Source: CAD feature listing. Evaluate the final solid. Frame: model axes, mm. Face numbers are marked on the shaded views. A direction names the side the tool comes from. Coordinates: 2 decimals unless noted, no trailing zeros. Loops run counter-clockwise (first coordinate to the right, second up) from the corner with the lowest first, then second, coordinate; pieces in that order, holes last.
Item 1: Reachability of the marked faces 1, 2, 3 and 4 from +Z, -Z, +X, -X, +Y, -Y: full face, straight path, thin tool, end or side. Return the list, or none.
Item 2: Section query A-A, the plane z = 19.5. Return the cut outline in (x, y).
Item 3: Line query: probe 1 along Z at (x, y) = (34.5, -25); probe 2 along X at (y, z) = (77, 20); probe 3 along X at (y, z) = (-0.5, 20.5). Output: solid intervals per line, ascending.
Item 4: Pin query (flat end, axial travel): pin 1 Ø6 at (y, z) = (73, 20.5) entering from -X; pin 2 Ø7.5 at (x, z) = (-9, 22.5) entering from -Y; pin 3 Ø5 at (y, z) = (-30.5, 9.5) entering from -X. Return the tip coordinate at first contact, or that it passes through.
Item 5: Section query B-B, the plane z = 2.5. Return the cut outline in (x, y), then the cut area to 3 significant figures.
Item 6: Pull-direction query (Y, two-part tool) for the marked faces 5, 6 and 7; classes: +Y half, -Y half, draft (parallel to the pull), parting line (faces both ways), or undercut.
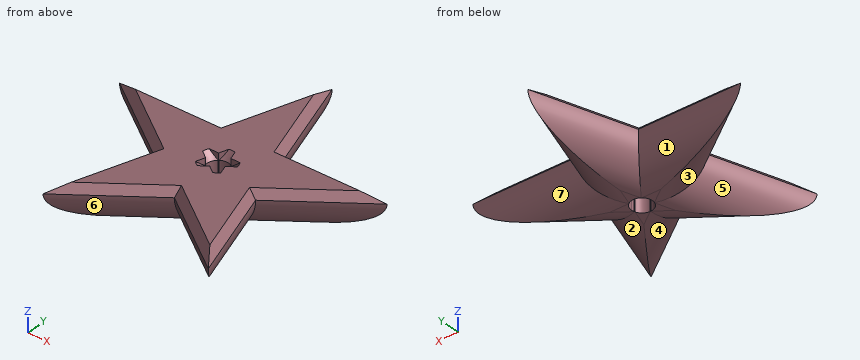
```python
from build123d import *

# Parameters (mm, degrees)
F1_DEPTH     = 30
F2_SIZE      = 5
F3_R         = 24.99999
F5_DEPTH     = 35
F6_T4_ANGLE  = 264.2993733481
F6_T11_ANGLE = 264.2993733481
F6_T18_ANGLE = 264.2993733481
F6_T24_ANGLE = 264.2993733481
F6_T30_ANGLE = 264.2993733481
F6_T37_ANGLE = 264.2993733481
F6_T44_ANGLE = 264.2993733481
F6_T51_ANGLE = 264.2993733481
F6_T57_ANGLE = 264.2993733481
F6_T63_ANGLE = 264.2993733481
F6_T70_ANGLE = 264.299373348
F6_T77_ANGLE = 264.299373348
F6_T84_ANGLE = 264.299373348


# Not quite as in the source:
# - a fillet or chamfer that OpenCascade refuses, or shapes differently, is made with other operations: its cross-section is extruded or revolved along the edge and cut away or added
# - a fillet or chamfer is up to 0.001 mm smaller than in the source, because OpenCascade refuses the exact size


with BuildPart() as f1:
    # F0 (on Top) → F1 (new body)
    with BuildSketch(Plane.XY):
        Polygon((22.451398829, 30.9016994375), (0, 100), (-22.451398829, 30.9016994375), (-95.1056516295, 30.9016994375), (-36.3271264003, -11.803398875), (-58.7785252292, -80.9016994375), (0, -38.196601125), (58.7785252292, -80.9016994375), (36.3271264003, -11.803398875), (95.1056516295, 30.9016994375), align=None)
    extrude(amount=F1_DEPTH)

    # F2
    f2_edges = [f1.edges().sort_by_distance(p)[0] for p in [
        (65.716389, 9.54915, 30),
        (58.778525, 30.901699, 30),
        (11.225699, 65.45085, 30),
        (-11.225699, 65.45085, 30),
        (-58.778525, 30.901699, 30),
        (-65.716389, 9.54915, 30),
        (-47.552826, -46.352549, 30),
        (-29.389263, -59.54915, 30),
        (29.389263, -59.54915, 30),
        (47.552826, -46.352549, 30),
    ]]
    chamfer(f2_edges, length=F2_SIZE)

    # F3 (radius 25 in the source; OpenCascade refuses exactly that, so slightly less here)
    f3_edges = [f1.edges().sort_by_distance(p)[0] for p in [
        (65.716389, 9.54915, 0),
        (58.778525, 30.901699, 0),
        (11.225699, 65.45085, 0),
        (-11.225699, 65.45085, 0),
        (-58.778525, 30.901699, 0),
        (-65.716389, 9.54915, 0),
        (-47.552826, -46.352549, 0),
        (-29.389263, -59.54915, 0),
        (29.389263, -59.54915, 0),
        (47.552826, -46.352549, 0),
    ]]
    fillet(f3_edges, radius=F3_R)

    # F4 (on face) → F5 (cut)
    with BuildSketch(Plane(origin=(0, 0, 0), x_dir=(1, 0, 0), z_dir=(0, 0, -1))):
        with BuildLine():
            ThreePointArc((4.6281557575, -5.9017094375), (6.7439294251, -3.2816788249), (7.5, 0))
            ThreePointArc((7.5, 0), (7.4279525521, 1.0370732295), (7.2131944311, 2.0542215312))
            Line((7.2131944311, 2.0542215312), (6.9378755413, 2.2542524134))
            Line((6.9378755413, 2.2542524134), (7.0430379995, 2.5779091795))
            ThreePointArc((7.0430379995, 2.5779091795), (4.4083893922, 6.0676274578), (0.2753188897, 7.4949449303))
            Line((0.2753188897, 7.4949449303), (0, 7.2949140482))
            Line((0, 7.2949140482), (-0.2753188897, 7.4949449303))
            ThreePointArc((-0.2753188897, 7.4949449303), (-4.4083893922, 6.0676274578), (-7.0430379995, 2.5779091795))
            Line((-7.0430379995, 2.5779091795), (-6.9378755413, 2.2542524134))
            Line((-6.9378755413, 2.2542524134), (-7.2131944311, 2.0542215312))
            ThreePointArc((-7.2131944311, 2.0542215312), (-7.1329238722, -2.3176274578), (-4.6281557575, -5.9017094375))
            Line((-4.6281557575, -5.9017094375), (-4.2878428943, -5.9017094375))
            Line((-4.2878428943, -5.9017094375), (-4.1826804361, -6.2253662036))
            ThreePointArc((-4.1826804361, -6.2253662036), (0, -7.5), (4.1826804361, -6.2253662036))
            Line((4.1826804361, -6.2253662036), (4.2878428943, -5.9017094375))
            Line((4.2878428943, -5.9017094375), (4.6281557575, -5.9017094375))
        make_face()
    extrude(amount=-F5_DEPTH, mode=Mode.SUBTRACT)

    # F6: chamfer of 5 on 5 edges, made by hand


with BuildPart() as f6_tool2:
    # F6_s3 → F6_t4 (revolve)
    with BuildSketch(Plane(origin=(0, 0, 0), x_dir=(0, 0, 1), z_dir=(0.9124797315, 0.4091219129, 0))):
        Polygon((30, 12.5), (25, 7.5), (30, 7.5), align=None)
    revolve(axis=Axis((0, 0, 30), (0, 0, -1)), revolution_arc=F6_T4_ANGLE)

    split(bisect_by=Plane(origin=(-5.6128592178, 1.823728512, 0), x_dir=(0, 0, 1), z_dir=(0.9510565163, -0.3090169944, 0)), keep=Keep.TOP)

    split(bisect_by=Plane(origin=(-3.4689377707, -4.7745832308, 0), x_dir=(0, 0, 1), z_dir=(0.5877852523, 0.8090169944, 0)), keep=Keep.TOP)

    split(bisect_by=Plane(origin=(5.6128592178, 1.823728512, 0), x_dir=(0, 0, 1), z_dir=(-0.9510565163, -0.3090169944, 0)), keep=Keep.TOP)


with BuildPart() as f1_1:
    add(f1.part)

    # F6_t1: cut F6_tool2
    add(f6_tool2.part, mode=Mode.SUBTRACT)


with BuildPart() as f6_tool9:
    # F6_s10 → F6_t11 (revolve)
    with BuildSketch(Plane(origin=(0, 0, 0), x_dir=(0, 0, 1), z_dir=(0.9124797315, 0.4091219129, 0))):
        Polygon((30, 12.5), (25, 7.5), (30, 7.5), align=None)
    revolve(axis=Axis((0, 0, 30), (0, 0, -1)), revolution_arc=F6_T11_ANGLE)

    split(bisect_by=Plane.XZ.offset(-5.9017094375), keep=Keep.TOP)

    split(bisect_by=Plane(origin=(-5.6128592178, 1.823728512, 0), x_dir=(0, 0, 1), z_dir=(0.9510565163, -0.3090169944, 0)), keep=Keep.TOP)

    split(bisect_by=Plane(origin=(3.4689377707, -4.7745832308, 0), x_dir=(0, 0, 1), z_dir=(-0.5877852523, 0.8090169944, 0)), keep=Keep.TOP)


with BuildPart() as f1_2:
    add(f1_1.part)

    # F6_t8: cut F6_tool9
    add(f6_tool9.part, mode=Mode.SUBTRACT)


with BuildPart() as f6_tool16:
    # F6_s17 → F6_t18 (revolve)
    with BuildSketch(Plane(origin=(0, 0, 0), x_dir=(0, 0, 1), z_dir=(0.9124797315, 0.4091219129, 0))):
        Polygon((30, 12.5), (25, 7.5), (30, 7.5), align=None)
    revolve(axis=Axis((0, 0, 30), (0, 0, -1)), revolution_arc=F6_T18_ANGLE)

    split(bisect_by=Plane.XZ.offset(-5.9017094375), keep=Keep.TOP)

    split(bisect_by=Plane(origin=(-3.4689377707, -4.7745832308, 0), x_dir=(0, 0, 1), z_dir=(0.5877852523, 0.8090169944, 0)), keep=Keep.TOP)


with BuildPart() as f1_3:
    add(f1_2.part)

    # F6_t15: cut F6_tool16
    add(f6_tool16.part, mode=Mode.SUBTRACT)


with BuildPart() as f6_tool22:
    # F6_s23 → F6_t24 (revolve)
    with BuildSketch(Plane(origin=(0, 0, 0), x_dir=(0, 0, 1), z_dir=(0.6710698053, -0.7413941707, 0))):
        Polygon((30, 12.5), (25, 7.5), (30, 7.5), align=None)
    revolve(axis=Axis((0, 0, 30), (0, 0, -1)), revolution_arc=F6_T24_ANGLE)

    split(bisect_by=Plane(origin=(5.6128592178, 1.823728512, 0), x_dir=(0, 0, 1), z_dir=(-0.9510565163, -0.3090169944, 0)), keep=Keep.TOP)

    split(bisect_by=Plane(origin=(-5.6128592178, 1.823728512, 0), x_dir=(0, 0, 1), z_dir=(0.9510565163, -0.3090169944, 0)), keep=Keep.TOP)


with BuildPart() as f1_4:
    add(f1_3.part)

    # F6_t21: cut F6_tool22
    add(f6_tool22.part, mode=Mode.SUBTRACT)


with BuildPart() as f6_tool28:
    # F6_s29 → F6_t30 (revolve)
    with BuildSketch(Plane(origin=(0, 0, 0), x_dir=(0, 0, 1), z_dir=(0.6710698053, -0.7413941707, 0))):
        Polygon((30, 12.5), (25, 7.5), (30, 7.5), align=None)
    revolve(axis=Axis((0, 0, 30), (0, 0, -1)), revolution_arc=F6_T30_ANGLE)

    split(bisect_by=Plane(origin=(3.4689377707, -4.7745832308, 0), x_dir=(0, 0, 1), z_dir=(-0.5877852523, 0.8090169944, 0)), keep=Keep.TOP)

    split(bisect_by=Plane.XZ.offset(-5.9017094375), keep=Keep.TOP)

    split(bisect_by=Plane(origin=(-3.4689377707, -4.7745832308, 0), x_dir=(0, 0, 1), z_dir=(0.5877852523, 0.8090169944, 0)), keep=Keep.TOP)


with BuildPart() as f1_5:
    add(f1_4.part)

    # F6_t27: cut F6_tool28
    add(f6_tool28.part, mode=Mode.SUBTRACT)


with BuildPart() as f6_tool35:
    # F6_s36 → F6_t37 (revolve)
    with BuildSketch(Plane(origin=(0, 0, 0), x_dir=(0, 0, 1), z_dir=(-0.497735783, -0.8673287095, 0))):
        Polygon((30, 12.5), (25, 7.5), (30, 7.5), align=None)
    revolve(axis=Axis((0, 0, 30), (0, 0, -1)), revolution_arc=F6_T37_ANGLE)

    split(bisect_by=Plane(origin=(5.6128592178, 1.823728512, 0), x_dir=(0, 0, 1), z_dir=(-0.9510565163, -0.3090169944, 0)), keep=Keep.TOP)

    split(bisect_by=Plane.XZ.offset(-5.9017094375), keep=Keep.TOP)

    split(bisect_by=Plane(origin=(-3.4689377707, -4.7745832308, 0), x_dir=(0, 0, 1), z_dir=(0.5877852523, 0.8090169944, 0)), keep=Keep.TOP)


with BuildPart() as f1_6:
    add(f1_5.part)

    # F6_t34: cut F6_tool35
    add(f6_tool35.part, mode=Mode.SUBTRACT)


with BuildPart() as f6_tool42:
    # F6_s43 → F6_t44 (revolve)
    with BuildSketch(Plane(origin=(0, 0, 0), x_dir=(0, 0, 1), z_dir=(-0.497735783, -0.8673287095, 0))):
        Polygon((30, 12.5), (25, 7.5), (30, 7.5), align=None)
    revolve(axis=Axis((0, 0, 30), (0, 0, -1)), revolution_arc=F6_T44_ANGLE)

    split(bisect_by=Plane(origin=(3.4689377707, -4.7745832308, 0), x_dir=(0, 0, 1), z_dir=(-0.5877852523, 0.8090169944, 0)), keep=Keep.TOP)

    split(bisect_by=Plane(origin=(5.6128592178, 1.823728512, 0), x_dir=(0, 0, 1), z_dir=(-0.9510565163, -0.3090169944, 0)), keep=Keep.TOP)

    split(bisect_by=Plane(origin=(-5.6128592178, 1.823728512, 0), x_dir=(0, 0, 1), z_dir=(0.9510565163, -0.3090169944, 0)), keep=Keep.TOP)


with BuildPart() as f1_7:
    add(f1_6.part)

    # F6_t41: cut F6_tool42
    add(f6_tool42.part, mode=Mode.SUBTRACT)


with BuildPart() as f6_tool49:
    # F6_s50 → F6_t51 (revolve)
    with BuildSketch(Plane(origin=(0, 0, 0), x_dir=(0, 0, 1), z_dir=(-0.497735783, -0.8673287095, 0))):
        Polygon((30, 12.5), (25, 7.5), (30, 7.5), align=None)
    revolve(axis=Axis((0, 0, 30), (0, 0, -1)), revolution_arc=F6_T51_ANGLE)

    split(bisect_by=Plane(origin=(3.4689377707, -4.7745832308, 0), x_dir=(0, 0, 1), z_dir=(-0.5877852523, 0.8090169944, 0)), keep=Keep.TOP)

    split(bisect_by=Plane.XZ.offset(-5.9017094375), keep=Keep.TOP)


with BuildPart() as f1_8:
    add(f1_7.part)

    # F6_t48: cut F6_tool49
    add(f6_tool49.part, mode=Mode.SUBTRACT)


with BuildPart() as f6_tool55:
    # F6_s56 → F6_t57 (revolve)
    with BuildSketch(Plane(origin=(0, 0, 0), x_dir=(0, 0, 1), z_dir=(-0.9786874366, 0.2053555488, 0))):
        Polygon((30, 12.5), (25, 7.5), (30, 7.5), align=None)
    revolve(axis=Axis((0, 0, 30), (0, 0, -1)), revolution_arc=F6_T57_ANGLE)

    split(bisect_by=Plane(origin=(5.6128592178, 1.823728512, 0), x_dir=(0, 0, 1), z_dir=(-0.9510565163, -0.3090169944, 0)), keep=Keep.TOP)

    split(bisect_by=Plane(origin=(-3.4689377707, -4.7745832308, 0), x_dir=(0, 0, 1), z_dir=(0.5877852523, 0.8090169944, 0)), keep=Keep.TOP)


with BuildPart() as f1_9:
    add(f1_8.part)

    # F6_t54: cut F6_tool55
    add(f6_tool55.part, mode=Mode.SUBTRACT)


with BuildPart() as f6_tool61:
    # F6_s62 → F6_t63 (revolve)
    with BuildSketch(Plane(origin=(0, 0, 0), x_dir=(0, 0, 1), z_dir=(-0.9786874366, 0.2053555488, 0))):
        Polygon((30, 12.5), (25, 7.5), (30, 7.5), align=None)
    revolve(axis=Axis((0, 0, 30), (0, 0, -1)), revolution_arc=F6_T63_ANGLE)

    split(bisect_by=Plane(origin=(3.4689377707, -4.7745832308, 0), x_dir=(0, 0, 1), z_dir=(-0.5877852523, 0.8090169944, 0)), keep=Keep.TOP)

    split(bisect_by=Plane.XZ.offset(-5.9017094375), keep=Keep.TOP)

    split(bisect_by=Plane(origin=(-5.6128592178, 1.823728512, 0), x_dir=(0, 0, 1), z_dir=(0.9510565163, -0.3090169944, 0)), keep=Keep.TOP)


with BuildPart() as f1_10:
    add(f1_9.part)

    # F6_t60: cut F6_tool61
    add(f6_tool61.part, mode=Mode.SUBTRACT)


with BuildPart() as f6_tool68:
    # F6_s69 → F6_t70 (revolve)
    with BuildSketch(Plane(origin=(0, 0, 0), x_dir=(0, 0, 1), z_dir=(-0.1071263172, 0.9942454185, 0))):
        Polygon((30, 12.5), (25, 7.5), (30, 7.5), align=None)
    revolve(axis=Axis((0, 0, 30), (0, 0, -1)), revolution_arc=F6_T70_ANGLE)

    split(bisect_by=Plane(origin=(3.4689377707, -4.7745832308, 0), x_dir=(0, 0, 1), z_dir=(-0.5877852523, 0.8090169944, 0)), keep=Keep.TOP)

    split(bisect_by=Plane(origin=(-3.4689377707, -4.7745832308, 0), x_dir=(0, 0, 1), z_dir=(0.5877852523, 0.8090169944, 0)), keep=Keep.TOP)

    split(bisect_by=Plane.XZ.offset(-5.9017094375), keep=Keep.TOP)


with BuildPart() as f1_11:
    add(f1_10.part)

    # F6_t67: cut F6_tool68
    add(f6_tool68.part, mode=Mode.SUBTRACT)


with BuildPart() as f6_tool75:
    # F6_s76 → F6_t77 (revolve)
    with BuildSketch(Plane(origin=(0, 0, 0), x_dir=(0, 0, 1), z_dir=(-0.1071263172, 0.9942454185, 0))):
        Polygon((30, 12.5), (25, 7.5), (30, 7.5), align=None)
    revolve(axis=Axis((0, 0, 30), (0, 0, -1)), revolution_arc=F6_T77_ANGLE)

    split(bisect_by=Plane(origin=(5.6128592178, 1.823728512, 0), x_dir=(0, 0, 1), z_dir=(-0.9510565163, -0.3090169944, 0)), keep=Keep.TOP)

    split(bisect_by=Plane(origin=(-5.6128592178, 1.823728512, 0), x_dir=(0, 0, 1), z_dir=(0.9510565163, -0.3090169944, 0)), keep=Keep.TOP)

    split(bisect_by=Plane(origin=(-3.4689377707, -4.7745832308, 0), x_dir=(0, 0, 1), z_dir=(0.5877852523, 0.8090169944, 0)), keep=Keep.TOP)


with BuildPart() as f1_12:
    add(f1_11.part)

    # F6_t74: cut F6_tool75
    add(f6_tool75.part, mode=Mode.SUBTRACT)


with BuildPart() as f6_tool82:
    # F6_s83 → F6_t84 (revolve)
    with BuildSketch(Plane(origin=(0, 0, 0), x_dir=(0, 0, 1), z_dir=(-0.1071263172, 0.9942454185, 0))):
        Polygon((30, 12.5), (25, 7.5), (30, 7.5), align=None)
    revolve(axis=Axis((0, 0, 30), (0, 0, -1)), revolution_arc=F6_T84_ANGLE)

    split(bisect_by=Plane(origin=(3.4689377707, -4.7745832308, 0), x_dir=(0, 0, 1), z_dir=(-0.5877852523, 0.8090169944, 0)), keep=Keep.TOP)

    split(bisect_by=Plane(origin=(-5.6128592178, 1.823728512, 0), x_dir=(0, 0, 1), z_dir=(0.9510565163, -0.3090169944, 0)), keep=Keep.TOP)


with BuildPart() as f1_13:
    add(f1_12.part)

    # F6_t81: cut F6_tool82
    add(f6_tool82.part, mode=Mode.SUBTRACT)


solid = f1_13.part
```
Verdict:
1. face 1: -Z, -X, +Y
1. face 2: -Z, +X
1. face 3: -Z, -X
1. face 4: -Z, -Y
2. outline: (-93.22, 30.29) - (-35.61, -11.57) - (-57.61, -79.3) - (0, -37.44) - (57.61, -79.3) - (35.61, -11.57) - (93.22, 30.29) - (22.01, 30.29) - (0, 98.02) - (-22.01, 30.29) - close; hole (-7.21, -2.05) - (-6.94, -2.25) - (-7.04, -2.58) arc R7.5 ccw to (-0.28, -7.49) - (0, -7.29) - (0.28, -7.49) arc R7.5 ccw to (7.04, -2.58) - (6.94, -2.25) - (7.21, -2.05) arc R7.5 ccw to (4.63, 5.9) - (4.29, 5.9) - (4.18, 6.23) arc R7.5 ccw to (-4.18, 6.23) - (-4.29, 5.9) - (-4.63, 5.9) arc R7.5 ccw to start
3. probe 1: z = 8.97 to 30
3. probe 2: x = -6.94 to 6.94
3. probe 3: x = -51.19 to -7.48, 7.48 to 51.19
4. pin 1: stops at x = -9.44
4. pin 2: stops at y = -47.34
4. pin 3: stops at x = -38.76
5. outline: (-51.7, 16.8) - (-19.75, -6.42) - (-31.95, -43.98) - (0, -20.76) - (31.95, -43.98) - (19.75, -6.42) - (51.7, 16.8) - (12.21, 16.8) - (0, 54.36) - (-12.21, 16.8) - close; hole (-7.21, -2.05) - (-6.94, -2.25) - (-7.04, -2.58) arc R7.5 ccw to (-0.28, -7.49) - (0, -7.29) - (0.28, -7.49) arc R7.5 ccw to (7.04, -2.58) - (6.94, -2.25) - (7.21, -2.05) arc R7.5 ccw to (4.63, 5.9) - (4.29, 5.9) - (4.18, 6.23) arc R7.5 ccw to (-4.18, 6.23) - (-4.29, 5.9) - (-4.63, 5.9) arc R7.5 ccw to start
5. area: 3,140 mm2
6. face 5: undercut
6. face 6: -Y half
6. face 7: +Y half
